Read the model definition and answer for the solid it produces. Units are mm, in the model's axes. Face numbers are marked on the shaded views. A direction names the side the tool comes from. Coordinates: 2 decimals unless noted, no trailing zeros. Write each loop counter-clockwise with the first axis right and the second up, starting at its lowest first coordinate (ties: lowest second). Pieces come first, ordered by that corner, then holes. Notation, with made-up numbers: (-5, -23) -> (-1, -23) arc R6 cw to (-1, -19) -> close; hole circle Ø10 at (5, 42). An arc over 180 degrees is marked (long way). Write item = value, one per line. Start each with the question number.
1) Section D-D (y = -15.5) is taken. Determine the outline of the cut face in (x, z).
2) For a pull along Y with two mould halves and no side action, classify the marked faces 5, 6 and 7 as released by +Y, released by -Y, zero draft, split by the parting line, or undercut.
3) Section A-A (y = 0) is taken. Determine the outline of the cut face in (x, z).
4) A tool of negligible diameter and unlimited length cuts with its end or side. For the marked faces 1, 2, 3 and 4, from which of +Z, -Z, +X, -X, +Y, -Y can it reach the whole face along a straight path? Write none if from no direction.
5) Flat-ended cylindrical pins translate along their axes: pin 1 Ø6 at (x, y) = (5.5, 26) entering from +Z; pin 2 Ø3 at (x, z) = (6.5, 23) entering from +Y (3 decimals); pin 3 Ø4 at (x, y) = (11.5, 6.5) entering from -Z. Find the tip coordinate at first contact, or state that the pin passes through.
6) Find the intervals of material crossed by line 1 along Z through (x, y) = (9.25, -29.5); line 2 along Z through (x, y) = (7.5, -36.5); line 3 along Y through (x, z) = (11, -7), in increasing order. Write a range as from..to.
7) Section C-C (z = -21.5) is taken. Determine the outline of the cut face in (x, y).
from build123d import *

# Parameters (mm, degrees)
BASPROSKE_W        = 15
BASPROSKE_H        = 44
TOOTHCUT_DEPTH     = 65.007812023
TEETHCUTS_DEPTH    = 15
BORSKE_R           = 3
BORE_DEPTH         = 50.0000508
CUT_EXTRUDE1_REACH = 65.743


# Read off the part's stored shape, not the designer's step: TeethCuts
with BuildPart() as part:
    # BasProSke → Base-Revolve (revolve)
    with BuildSketch(Plane(origin=(0, 0, 0), x_dir=(1, 0, 0), z_dir=(0, 1, 0)), mode=Mode.PRIVATE) as base_revolve_sk:
        with Locations((7.5, 22)):
            Rectangle(BASPROSKE_W, BASPROSKE_H)
    revolve(base_revolve_sk.sketch.rotate(Axis((-10, 0, 0), (1, 0, 0)), 180), axis=Axis((-10, 0, 0), (1, 0, 0)))

    # TooCutSke → ToothCut (cut, through all)
    with BuildSketch(Plane(origin=(0, 0, 0), x_dir=(0, 0, -1), z_dir=(1, 0, 0))):
        with BuildLine():
            ThreePointArc((1.961730392, 34.943978235), (0, 34.999), (-1.961730392, 34.943978235))
            ThreePointArc((-1.961730392, 34.943978235), (-3.235659864, 39.585086827), (-5.832115241, 43.637395396))
            ThreePointArc((-5.832115241, 43.637395396), (0, 44.0254), (5.832115241, 43.637395396))
            ThreePointArc((5.832115241, 43.637395396), (3.235659864, 39.585086827), (1.961730392, 34.943978235))
        make_face()
    extrude(amount=TOOTHCUT_DEPTH, mode=Mode.SUBTRACT)

    # TeethCuts outline → TeethCuts (cut)
    with BuildSketch(Plane.YZ):
        with BuildLine():
            ThreePointArc((39.683804298, 19.005148682), (36.636439054, 15.299557845), (32.627490176, 12.663999598))
            ThreePointArc((32.627490176, 12.663999598), (33.286027014, 10.815285786), (33.839906235, 8.932566653))
            ThreePointArc((33.839906235, 8.932566653), (38.632356276, 9.156756269), (43.275818192, 7.950066657))
            ThreePointArc((43.275818192, 7.950066657), (41.846486717, 13.596747753), (39.683804298, 19.005148682))
        make_face()
        with BuildLine():
            ThreePointArc((-34.943978235, 1.961730392), (-39.571147477, 3.229461904), (-43.614454593, 5.812000568))
            ThreePointArc((-43.614454593, 5.812000568), (-44, 0), (-43.614454592, -5.812000568))
            ThreePointArc((-43.614454592, -5.812000568), (-39.571147477, -3.229461904), (-34.943978235, -1.961730392))
            ThreePointArc((-34.943978235, -1.961730392), (-34.999, 0), (-34.943978235, 1.961730392))
        make_face()
        with BuildLine():
            ThreePointArc((-32.627490176, 12.663999598), (-36.636439054, 15.299557845), (-39.683804298, 19.005148682))
            ThreePointArc((-39.683804298, 19.005148682), (-41.846486717, 13.596747753), (-43.275818192, 7.950066657))
            ThreePointArc((-43.275818192, 7.950066657), (-38.632356276, 9.156756269), (-33.839906235, 8.932566653))
            ThreePointArc((-33.839906235, 8.932566653), (-33.286027014, 10.815285786), (-32.627490176, 12.663999598))
        make_face()
        with BuildLine():
            ThreePointArc((-27.117196049, 22.126628289), (-30.115500715, 25.872026467), (-31.868626746, 30.337940427))
            ThreePointArc((-31.868626746, 30.337940427), (-35.596747753, 25.862551101), (-38.701043186, 20.933925966))
            ThreePointArc((-38.701043186, 20.933925966), (-33.911960876, 20.64664734), (-29.423348436, 18.952481837))
            ThreePointArc((-29.423348436, 18.952481837), (-28.314785786, 20.571896045), (-27.117196049, 22.126628289))
        make_face()
        with BuildLine():
            ThreePointArc((-18.952481837, 29.423348436), (-20.64664734, 33.911960876), (-20.933925966, 38.701043186))
            ThreePointArc((-20.933925966, 38.701043186), (-25.862551101, 35.596747753), (-30.337940427, 31.868626746))
            ThreePointArc((-30.337940427, 31.868626746), (-25.872026467, 30.115500715), (-22.126628289, 27.117196049))
            ThreePointArc((-22.126628289, 27.117196049), (-20.571896045, 28.314785786), (-18.952481837, 29.423348436))
        make_face()
        with BuildLine():
            ThreePointArc((-8.932566653, 33.839906235), (-9.156756269, 38.632356276), (-7.950066657, 43.275818192))
            ThreePointArc((-7.950066657, 43.275818192), (-13.596747753, 41.846486717), (-19.005148682, 39.683804298))
            ThreePointArc((-19.005148682, 39.683804298), (-15.299557845, 36.636439054), (-12.663999598, 32.627490176))
            ThreePointArc((-12.663999598, 32.627490176), (-10.815285786, 33.286027014), (-8.932566653, 33.839906235))
        make_face()
        with BuildLine():
            ThreePointArc((1.961730392, 34.943978235), (3.229461904, 39.571147477), (5.812000568, 43.614454593))
            ThreePointArc((5.812000568, 43.614454593), (0, 44), (-5.812000568, 43.614454593))
            ThreePointArc((-5.812000568, 43.614454593), (-3.229461904, 39.571147477), (-1.961730392, 34.943978235))
            ThreePointArc((-1.961730392, 34.943978235), (0, 34.999), (1.961730392, 34.943978235))
        make_face()
        with BuildLine():
            ThreePointArc((12.663999598, 32.627490176), (15.299557845, 36.636439054), (19.005148682, 39.683804298))
            ThreePointArc((19.005148682, 39.683804298), (13.596747753, 41.846486717), (7.950066657, 43.275818192))
            ThreePointArc((7.950066657, 43.275818192), (9.156756269, 38.632356276), (8.932566653, 33.839906235))
            ThreePointArc((8.932566653, 33.839906235), (10.815285786, 33.286027014), (12.663999598, 32.627490176))
        make_face()
        with BuildLine():
            ThreePointArc((22.126628289, 27.117196049), (25.872026467, 30.115500715), (30.337940427, 31.868626746))
            ThreePointArc((30.337940427, 31.868626746), (25.862551101, 35.596747753), (20.933925966, 38.701043186))
            ThreePointArc((20.933925966, 38.701043186), (20.64664734, 33.911960876), (18.952481837, 29.423348436))
            ThreePointArc((18.952481837, 29.423348436), (20.571896045, 28.314785786), (22.126628289, 27.117196049))
        make_face()
        with BuildLine():
            ThreePointArc((29.423348436, 18.952481837), (33.911960876, 20.64664734), (38.701043186, 20.933925966))
            ThreePointArc((38.701043186, 20.933925966), (35.596747753, 25.862551101), (31.868626746, 30.337940427))
            ThreePointArc((31.868626746, 30.337940427), (30.115500715, 25.872026467), (27.117196049, 22.126628289))
            ThreePointArc((27.117196049, 22.126628289), (28.314785786, 20.571896045), (29.423348436, 18.952481837))
        make_face()
    extrude(amount=TEETHCUTS_DEPTH, mode=Mode.SUBTRACT)

    # BorSke → Bore (cut, symmetric)
    with BuildSketch(Plane(origin=(0, 0, 0), x_dir=(0, 0, -1), z_dir=(1, 0, 0))):
        with Locations(Location((0, 0, 0), (0, 0, 180))):
            Circle(BORSKE_R)
    extrude(amount=BORE_DEPTH, both=True, mode=Mode.SUBTRACT)

    # Sketch2 → Cut-Extrude1 (cut, up to next)
    with BuildSketch(Plane(origin=(15, 0, 0), x_dir=(0, 0, -1), z_dir=(1, 0, 0)), mode=Mode.PRIVATE) as cut_extrude1_sk1:
        with BuildLine():
            Line((1.961730392, -34.943978235), (2.123495302, -44.219744966))
            ThreePointArc((2.123495302, -44.219744966), (44.2706282, 0.080968685), (1.961730392, 44.227216632))
            Line((1.961730392, 44.227216632), (1.961730392, 34.943978235))
            ThreePointArc((1.961730392, 34.943978235), (34.999, 0), (1.961730392, -34.943978235))
        make_face()
    cut_extrude1_tool1 = extrude(cut_extrude1_sk1.sketch, amount=-CUT_EXTRUDE1_REACH, mode=Mode.PRIVATE) & part.part
    add(cut_extrude1_tool1.solids().sort_by_distance((15, 39.585597, -2.942185))[0], mode=Mode.SUBTRACT)


solid = part.part
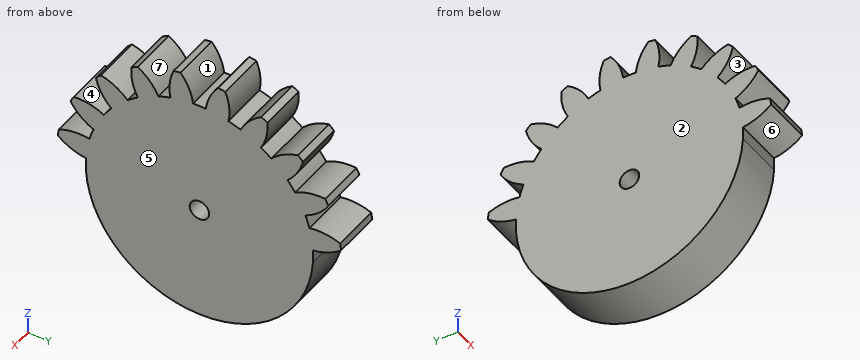
Answer key:
q1.outline = (0, -31.38) -> (15, -31.38) -> (15, 36.86) -> (0, 36.86) -> close
q2.face_5 = zero draft
q2.face_6 = released by -Y
q2.face_7 = undercut
q3.outline = (0, -35) -> (15, -35) -> (15, -3) -> (0, -3) -> close; (0, 3) -> (15, 3) -> (15, 35) -> (0, 35) -> close
q4.face_1 = +Z, +X, -X
q4.face_2 = +Z, -Z, -X, +Y, -Y
q4.face_3 = +X, -X, -Y
q4.face_4 = +X, -X
q5.pin_1 = 31.5
q5.pin_2 = 29.225
q5.pin_3 = -34.71
q6.line_1 = -18.83..19, 24.89..31.65
q6.line_2 = 2.22..9.24, 15.18..20.98
q6.line_3 = -34.29..34.29
q7.outline = (0, -27.62) -> (15, -27.62) -> (15, 27.62) -> (0, 27.62) -> close
